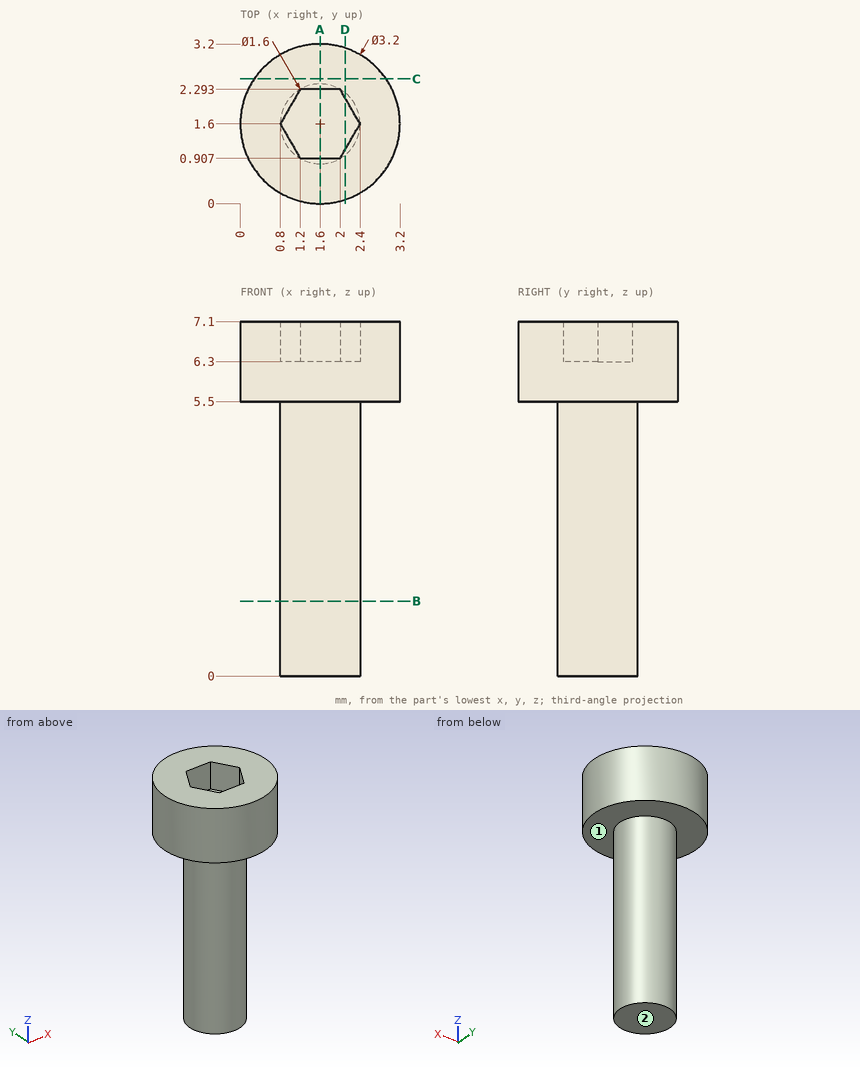
Drawing for the job (mm, zero at the part's lowest x, y, z). A direction names the side the tool comes from. Round coordinates to 2 decimals unless told otherwise and drop trailing zeros. Loops run counter-clockwise (first coordinate to the right, second up) from the corner with the lowest first, then second, coordinate; pieces in that order, holes last. Notation, with made-up numbers: (-15.75, 17.25) -> (25.25, 17.25) arc R15 ccw to (25.25, 41.25) -> close; hole circle Ø5 at (62.25, -12.5). An arc over 180 degrees is marked (long way). Answer as CSV lines item,"result". Start each with the question number.
1) Slice it at A-A (x = 1.6). List the corners of the cut face in (y, z).
2) Slice it at C-C (y = 2.5). List the corners of the cut face in (x, z).
3) Slice it at B-B (z = 1.5). List the corners of the cut face in (x, y).
4) Slice it at D-D (x = 2.1). List the corners of the cut face in (y, z), plus the area to 3 significant figures.
5) Tool access for the marked faces 1 and 2: list every direction of +Z, -Z, +X, -X, +Y, -Y with a clear straight run to the whole face (end or side of a thin tool).
6) Probe line 1 along Z through (x, y) = (1.65, 1.9); line 2 along X through (y, z) = (2, 1.5); line 3 along Z through (x, y) = (1.75, 2.8). List the from-to ranges inside material, lowest first.
Filled in:
1,outline,"(0, 5.5) -> (0.8, 5.5) -> (0.8, 0) -> (2.4, 0) -> (2.4, 5.5) -> (3.2, 5.5) -> (3.2, 7.1) -> (2.29, 7.1) -> (2.29, 6.3) -> (0.91, 6.3) -> (0.91, 7.1) -> (0, 7.1) -> close"
2,outline,"(0.28, 5.5) -> (2.92, 5.5) -> (2.92, 7.1) -> (0.28, 7.1) -> close"
3,outline,"circle Ø1.6 at (1.6, 1.6)"
4,outline,"(0.08, 5.5) -> (0.98, 5.5) -> (0.98, 0) -> (2.22, 0) -> (2.22, 5.5) -> (3.12, 5.5) -> (3.12, 7.1) -> (2.12, 7.1) -> (2.12, 6.3) -> (1.08, 6.3) -> (1.08, 7.1) -> (0.08, 7.1) -> close"
4,area,"10.9 mm2"
5,face 1,"-Z"
5,face 2,"-Z, +X, -X, +Y, -Y"
6,line 1,"z = 0 to 6.3"
6,line 2,"x = 0.91 to 2.29"
6,line 3,"z = 5.5 to 7.1"
